Autodesk Inventor part; units mm, degrees
ref_plane "to_ring_F_R_XY" through (17.575, 0, 0) normal (1, 0, 0) x (0, 0, -1)
ref_plane "to_ring_F_R_YZ" through (17.575, 0, 0) normal (0, 0, -1) x (0, 1, 0)
ref_plane "to_ring_F_R_ZX" through (17.575, 0, 0) normal (0, 1, 0) x (1, 0, 0)
sketch "Sketch_1" plane through (0, 0, 0) normal (0, 0, 1) x (1, 0, 0)
  line L0 (20, 0) -> (0, 0)
  line L1 (0, 0) -> (0, 4.5)
  line L2 (0, 4.5) -> (0.5, 5)
  line L3 (0.5, 5) -> (19.5, 5)
  line L4 (19.5, 5) -> (20, 4.5)
  line L5 (20, 4.5) -> (20, 0)
  line L6 (20, 0) -> (0, 0)
revolve "Revolution1" add sketch "Sketch_1" angle 360 about axis through (20, 0, 0) along (1, 0, 0)
sketch "Sketch2" plane through (0, 0, 0) normal (-1, 0, 0) x (0, 0, 1)
  point P0 (0, 0)
hole "Hole1" at (0, 0, 0) direction (1, 0, 0) diameter 4.134 depth 13.8066 tip angle 120 countersink diameter 5 countersink angle 90
sketch "Sketch_20" plane through (0, 0, 0) normal (0, 0, 1) x (1, 0, 0)
  line L0 (20, 0) -> (-20, 0)
  line L1 (17, 9.6) -> (17, 4.8)
  line L2 (17, 4.8) -> (18.15, 4.8)
  line L3 (18.15, 4.8) -> (18.15, 9.6)
  line L4 (18.15, 9.6) -> (17, 9.6)
revolve "Revolution2" cut sketch "Sketch_20" angle 360 about axis through (20, 0, 0) along (1, 0, 0)
ref_plane "to_ring_F_R_XY" through (17.575, 0, 0) normal (1, 0, 0) x (0, 0, -1)
ref_plane "to_ring_F_R_YZ" through (17.575, 0, 0) normal (0, 0, -1) x (0, 1, 0)
ref_plane "to_ring_F_R_ZX" through (17.575, 0, 0) normal (0, 1, 0) x (1, 0, 0)
properties part number "SSFRBF-D10-L20-M5-U3"
The model under review builds one solid part; all positions refer to its coordinate system, in mm. Coordinates: 2 decimals unless noted, no trailing zeros. Order: outer loops, then holes, each group sorted by start corner. A loop starts at its lowest first (then second) coordinate and runs counter-clockwise, first axis right, second up. Notation, with made-up numbers: (-16, 52) -> (18, 52) arc R12 ccw to (18, 59) -> close; hole circle Ø7 at (14, -19). An arc over 180 degrees is marked (long way). Answer in a Markdown table with one row per item. Add a question column.
Item 1: Mouldability with a two-part tool opening along Y and no side actions: class faces 1 (the flat face through (0, 2, -2)), 2 (the cylindrical face through (17.58, 2.58, 4.05)), 3 (the cylindrical face through (7.21, 1.26, -1.64)) as +Y half, -Y half, draft (parallel to the pull), parting line (faces both ways), or undercut.
Item 2: To check wall thickness, follow probe 1 along Z at (x, y) = (10, 0); probe 2 along Y at (x, z) = (9.25, 1.5); probe 3 along Y at (x, z) = (3, -1). State the ranges of each line that lie inside material, in increasing order.
Item 3: We need section B-B on x = 14.5. Write out the cut boundary in (y, z).
Item 4: We need section A-A on x = 6.25. Write out the cut boundary in (y, z), plus the area to 3 significant figures.
Item 5: Clearance check with flat-ended pins moving along their axes: pin 1 (4 mm diameter, centred on x = 17, y = 2.5, fed in from -Z); pin 2 (1.5 mm diameter, centred on x = 9.5, y = -0.5, fed in from +Z); pin 3 (1.5 mm diameter, centred on x = 8.5, z = 2.5, fed in from -Y). State where each tip first meets the part, or that it passes through.
Final values:
| question | item | result |
|---|---|---|
| 1 | face 1 | draft |
| 1 | face 2 | parting line |
| 1 | face 3 | undercut |
| 2 | probe 1 | z = -5 to -2.07, 2.07 to 5 |
| 2 | probe 2 | y = -4.77 to -1.42, 1.42 to 4.77 |
| 2 | probe 3 | y = -4.9 to -1.81, 1.81 to 4.9 |
| 3 | outline | circle Ø10 at (0, 0); hole circle Ø1.73 at (0, 0) |
| 4 | outline | circle Ø10 at (0, 0); hole circle Ø4.13 at (0, 0) |
| 4 | area | 65.1 mm2 |
| 5 | pin 1 | stops at z = -4.97 |
| 5 | pin 2 | stops at z = 5 |
| 5 | pin 3 | stops at y = -4.68 |
